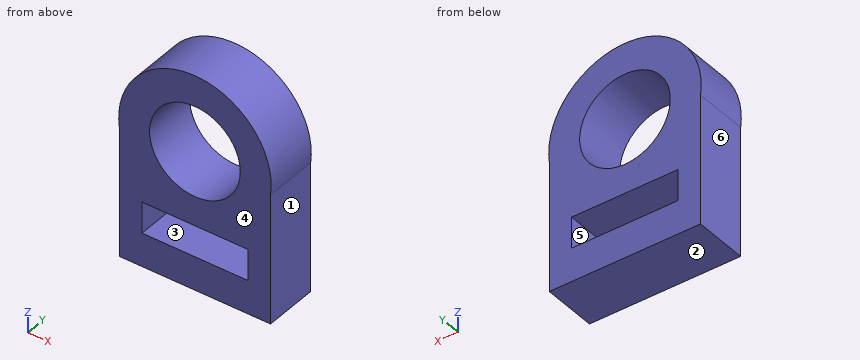
```python
from build123d import *

# Parameters (mm, degrees)
F0_W     = 49.235915
F0_H     = 14.462238
F0_R     = 21.012686
F1_DEPTH = 25


with BuildPart() as f1:
    # F0 (on Front) → F1 (new body)
    with BuildSketch(Plane.XZ):
        with BuildLine():
            ThreePointArc((70.080705, 0), (35.040352, 39.844464), (0, 0))
            Line((0, 0), (0, -60.007501))
            Line((0, -60.007501), (70.080705, -60.007501))
            Line((70.080705, -60.007501), (70.080705, 0))
        make_face()
        with Locations((35.122868, -37.23487)):
            Rectangle(F0_W, F0_H, mode=Mode.SUBTRACT)
        with Locations((35.040352, 4.514492)):
            Circle(F0_R, mode=Mode.SUBTRACT)
    extrude(amount=F1_DEPTH)


solid = f1.part
```
Check sheet for the modelled part. Datum: model origin and axes. Units: mm. Face numbers are marked on the shaded views. A direction names the side the tool comes from. Coordinates: 2 decimals unless noted, no trailing zeros. Write each loop counter-clockwise with the first axis right and the second up, starting at its lowest first coordinate (ties: lowest second). Pieces come first, ordered by that corner, then holes. Notation, with made-up numbers: M 3.5,53.25 L 51.5,53.25 A25 cw 51.5,81.25 Z; hole C -30.75,45.5 d8. An arc over 180 degrees is marked long. Write item = value, one per line. Start each with the question number.
1. Go/stop test with flat-tipped pins: pin 1 (12 mm diameter, centred on x = 13, y = -7.5, fed in from +Z); pin 2 (1.5 mm diameter, centred on y = -16.5, z = -46, fed in from -X); pin 3 (2 mm diameter, centred on x = 35.5, y = -6, fed in from +Z); pin 4 (3 mm diameter, centred on y = -19.5, z = 8.5, fed in from +X). Record where each tip stops, or that it passes through.
2. Sectioned sample at A-A (x = 40.5). Record the cut outline in (y, z), then the cut area to 3 significant figures.
3. Thickness scan on probe 1 along Z at (x, y) = (32, -4.25); probe 2 along Z at (x, y) = (29.5, -15.25); probe 3 along X at (y, z) = (-8.25, -33). Record the ranges inside material, lowest first.
4. Sectioned sample at B-B (z = 1). Record the cut outline in (x, y), then the cut area to 3 significant figures.
5. Mould release check, pull along X, two halves, no side actions. Record for the marked faces 4, 5 and 6: pulls with the +X half, pulls with the -X half, needs draft (parallel to the pull), parting line crosses it, or undercut.
6. Sectioned sample at D-D (x = 55). Record the cut outline in (y, z).
7. Sectioned sample at C-C (y = -20.5). Record the cut outline in (x, z), then the cut area to 4 significant figures.
8. Tool access check on the marked faces 1, 2 and 3. Record the directions out of +Z, -Z, +X, -X, +Y, -Y that give a thin tool (end or side, any length) a straight path to the whole face; none if there is none.
The answers:
q1.pin_1 = 35.99
q1.pin_2 = 0
q1.pin_3 = 39.84
q1.pin_4 = 70.28
q2.outline = M -25,-60.01 L 0,-60.01 L 0,-44.47 L -25,-44.47 Z; M -25,-30 L 0,-30 L 0,-15.78 L -25,-15.78 Z; M -25,24.81 L 0,24.81 L 0,39.42 L -25,39.42 Z
q2.area = 1,110 mm²
q3.probe_1 = -60.01 to -44.47, -30 to -16.28, 25.31 to 39.71
q3.probe_2 = -60.01 to -44.47, -30 to -15.75, 24.78 to 39.41
q3.probe_3 = 0 to 10.5, 59.74 to 70.08
q4.outline = M -0.11,-25 L 14.32,-25 L 14.32,0 L -0.11,0 Z; M 55.76,-25 L 70.2,-25 L 70.2,0 L 55.76,0 Z
q4.area = 722 mm²
q5.face_4 = needs draft
q5.face_5 = undercut
q5.face_6 = pulls with the -X half
q6.outline = M -25,-60.01 L 0,-60.01 L 0,-44.47 L -25,-44.47 Z; M -25,-30 L 0,-30 L 0,-2.05 L -25,-2.05 Z; M -25,11.08 L 0,11.08 L 0,33.67 L -25,33.67 Z
q7.outline = M 0,-60.01 L 70.08,-60.01 L 70.08,0 A35.33 ccw long 0,0 Z; hole M 10.5,-44.47 L 59.74,-44.47 L 59.74,-30 L 10.5,-30 Z; hole C 35.04,4.51 d42.03
q7.area = 4,385 mm²
q8.face_1 = -Z, +X, +Y, -Y
q8.face_2 = -Z, +X, -X, +Y, -Y
q8.face_3 = +Y, -Y
